CAD build for the part. Positions are in the model's coordinates, mm. Round coordinates to 2 decimals unless told otherwise and drop trailing zeros. Order: outer loops, then holes, each group sorted by start corner. A loop starts at its lowest first (then second) coordinate and runs counter-clockwise, first axis right, second up. Notation, with made-up numbers: (13.25, 28.5) -> (58.25, 28.5) arc R11 cw to (58.25, 48.5) -> close; hole circle Ø3 at (11.25, -36.75). An arc over 180 degrees is marked (long way). Return JSON: item names as keys, results as strings. Group by question number.
Q1. Cut at B-B (z = 6.75). Count the separate pieces of the cut face and the enclosed holes in it, then the cut area to 3 significant figures.
Q2. Cut at A-A (x = -22). Write the cut outline in (y, z).
Q3. Cut at C-C (x = 20). Write the cut outline in (y, z).
Q4. Probe line 1 along Y through (x, z) = (-13, 3); line 2 along Y through (x, z) = (-30.5, 6.25); line 3 along X through (y, z) = (0.5, 4.75). List the from-to ranges inside material, lowest first.
Q5. Mould opens along Y. For faces 1 (the cylindrical face through (-58.43, -1.37, 3.88)), 2 (the cylindrical face through (-15.117, -1.984, 3.885)), 3 (the flat face through (-29.6, 0.4, 0)), 4 (the cylindrical face through (-87.312, -4.731, 3.885)) say: +Y half, -Y half, draft (parallel to the pull), parting line (faces both ways), or undercut.
from build123d import *

# Parameters (mm, degrees)
F0_R        = 2.4
F1_DEPTH    = 7.88
F2_T1_DEPTH = 26.405


# Not quite as in the source:
# - a fillet or chamfer that OpenCascade refuses, or shapes differently, is made with other operations: its cross-section is extruded or revolved along the edge and cut away or added


with BuildPart() as f1:
    # F0 (on Top) → F1 (new body)
    with BuildSketch(Plane.XY):
        Polygon((30.9904916829, 1.6058013724), (-28.7195083171, 1.6058013724), (-88.4295083171, 1.6058013724), (-88.4295083171, -2.0891986276), (-88.4295083171, -5.7841986276), (-28.7195083171, -5.7841986276), (30.9904916829, -5.7841986276), (30.9904916829, -2.0891986276), align=None)
        with Locations((-84.7195083171, -2.0891986276)):
            Circle(F0_R, mode=Mode.SUBTRACT)
        with Locations((-76.7195083171, -2.0891986276)):
            Circle(F0_R, mode=Mode.SUBTRACT)
        with Locations((-68.7195083171, -2.0891986276)):
            Circle(F0_R, mode=Mode.SUBTRACT)
        with Locations((-60.7195083171, -2.0891986276)):
            Circle(F0_R, mode=Mode.SUBTRACT)
        with Locations((-52.7195083171, -2.0891986276)):
            Circle(F0_R, mode=Mode.SUBTRACT)
        with Locations((-44.7195083171, -2.0891986276)):
            Circle(F0_R, mode=Mode.SUBTRACT)
        with Locations((-36.7195083171, -2.0891986276)):
            Circle(F0_R, mode=Mode.SUBTRACT)
        with BuildLine():
            ThreePointArc((-28.7195083171, -4.4891986276), (-31.1195083171, -2.0891986276), (-28.7195083171, 0.3108013724))
            ThreePointArc((-28.7195083171, 0.3108013724), (-26.3195083171, -2.0891986276), (-28.7195083171, -4.4891986276))
        make_face(mode=Mode.SUBTRACT)
        with Locations((-20.7195083171, -2.0891986276)):
            Circle(F0_R, mode=Mode.SUBTRACT)
        with Locations((-12.7195083171, -2.0891986276)):
            Circle(F0_R, mode=Mode.SUBTRACT)
        with Locations((-4.7195083171, -2.0891986276)):
            Circle(F0_R, mode=Mode.SUBTRACT)
        with Locations((3.2804916829, -2.0891986276)):
            Circle(F0_R, mode=Mode.SUBTRACT)
        with Locations((11.2804916829, -2.0891986276)):
            Circle(F0_R, mode=Mode.SUBTRACT)
        with Locations((19.2804916829, -2.0891986276)):
            Circle(F0_R, mode=Mode.SUBTRACT)
        with Locations((27.2804916829, -2.0891986276)):
            Circle(F0_R, mode=Mode.SUBTRACT)
    extrude(amount=F1_DEPTH)

    # F2: fillet of radius 3.705 on 4 edges, made by hand

    # F2_s2 → F2_t1 (cut)
    with BuildSketch(Plane.XY.offset(-9.2625)):
        with BuildLine():
            ThreePointArc((27.2854916829, 1.6058013724), (29.9053223072, 0.5206319967), (30.9904916829, -2.0991986276))
            Line((30.9904916829, -2.0991986276), (30.9904916829, 1.6058013724))
            Line((30.9904916829, 1.6058013724), (27.2854916829, 1.6058013724))
        make_face()
        with BuildLine():
            ThreePointArc((27.2854916829, -5.7841986276), (29.9053223072, -4.6990292519), (30.9904916829, -2.0791986276))
            Line((30.9904916829, -2.0791986276), (30.9904916829, -5.7841986276))
            Line((30.9904916829, -5.7841986276), (27.2854916829, -5.7841986276))
        make_face()
        with BuildLine():
            ThreePointArc((-84.7245083171, 1.6058013724), (-87.3443389413, 0.5206319967), (-88.4295083171, -2.0991986276))
            Line((-88.4295083171, -2.0991986276), (-88.4295083171, 1.6058013724))
            Line((-88.4295083171, 1.6058013724), (-84.7245083171, 1.6058013724))
        make_face()
        with BuildLine():
            ThreePointArc((-84.7245083171, -5.7841986276), (-87.3443389413, -4.6990292519), (-88.4295083171, -2.0791986276))
            Line((-88.4295083171, -2.0791986276), (-88.4295083171, -5.7841986276))
            Line((-88.4295083171, -5.7841986276), (-84.7245083171, -5.7841986276))
        make_face()
    extrude(amount=F2_T1_DEPTH, mode=Mode.SUBTRACT)


solid = f1.part
Solution:
{
 "1": {"separate pieces": "1", "enclosed holes": "15", "area": "599 mm²"},
 "2": {"outline": "(-5.78, 0) -> (-4.12, 0) -> (-4.12, 7.88) -> (-5.78, 7.88) -> close; (-0.06, 0) -> (1.61, 0) -> (1.61, 7.88) -> (-0.06, 7.88) -> close"},
 "3": {"outline": "(-5.78, 0) -> (-4.38, 0) -> (-4.38, 7.88) -> (-5.78, 7.88) -> close; (0.2, 0) -> (1.61, 0) -> (1.61, 7.88) -> (0.2, 7.88) -> close"},
 "4": {"line 1": "y = -5.78 to -4.47, 0.29 to 1.61", "line 2": "y = -5.78 to -3.7, -0.48 to 1.61", "line 3": "x = -87.36 to 29.93"},
 "5": {"face 1": "undercut", "face 2": "undercut", "face 3": "draft", "face 4": "-Y half"}
}
